```python
from build123d import *

# Parameters (mm, degrees)
F0_W     = 395
F0_H     = 121
F1_DEPTH = 35.5
F2_W     = 120
F2_H     = 120
F3_DEPTH = 33
F4_R     = 10.191795
F5_DEPTH = 10
F6_R     = 2.5
F7_DEPTH = 10


with BuildPart() as f1:
    # F0 (on Right) → F1 (new body)
    with BuildSketch(Plane.YZ):
        Rectangle(F0_W, F0_H)
    extrude(amount=F1_DEPTH)

    # F2 (on face) → F3 (join)
    with BuildSketch(Plane(origin=(0, 0, 0), x_dir=(0, -1, 0), z_dir=(-1, 0, 0))):
        with Locations((-134.5, 0)):
            Rectangle(F2_W, F2_H)
        with Locations((-11.5, 0)):
            Rectangle(F2_W, F2_H)
        with Locations((111.5, 0)):
            Rectangle(F2_W, F2_H)
    extrude(amount=F3_DEPTH)

    # F4 (on face) → F5 (join)
    with BuildSketch(Plane(origin=(0, 0, 0), x_dir=(0, -1, 0), z_dir=(-1, 0, 0))):
        with Locations((185, 45)):
            Circle(F4_R)
        with Locations((185, -45)):
            Circle(F4_R)
    extrude(amount=F5_DEPTH)

    # F6 (on face) → F7 (cut)
    with BuildSketch(Plane.YZ.offset(35.5)):
        with Locations((180.5, -52.5)):
            Circle(F6_R)
        with Locations((75.5, -52.5)):
            Circle(F6_R)
        with Locations((60.5, -52.5)):
            Circle(F6_R)
        with Locations((180.5, 52.5)):
            Circle(F6_R)
        with Locations((75.5, 52.5)):
            Circle(F6_R)
        with Locations((60.5, 52.5)):
            Circle(F6_R)
        with Locations((-44.5, 52.5)):
            Circle(F6_R)
        with Locations((-59.5, 52.5)):
            Circle(F6_R)
        with Locations((-164.5, 52.5)):
            Circle(F6_R)
        with Locations((-44.5, -52.5)):
            Circle(F6_R)
        with Locations((-164.5, -52.5)):
            Circle(F6_R)
        with Locations((-59.5, -52.5)):
            Circle(F6_R)
    extrude(amount=-F7_DEPTH, mode=Mode.SUBTRACT)


solid = f1.part
```
Geometry check sheet. Reference: the model listing, model coordinates, mm. A direction names the side the tool comes from. Round coordinates to 2 decimals unless told otherwise and drop trailing zeros. Loops run counter-clockwise (first coordinate to the right, second up) from the corner with the lowest first, then second, coordinate; pieces in that order, holes last. Notation, with made-up numbers: (0.5, -16) - (5.5, -16) arc R24 ccw to (5.5, 15) - close; hole circle Ø4 at (84, 57). An arc over 180 degrees is marked (long way). Write item = value, one per line. Start each with the question number.
1. Set-up check for faces 1 (the face through (-16, 71.5, -1)), 2 (the face through (-10, -185, -45)), 3 (the face through (-4.93, -174.82, -44.55)): record each of +Z, -Z, +X, -X, +Y, -Y from which the full face is reachable in a straight line by a thin tool's end or side.
2. Depth check by flat-ended pin: pin 1 (2.5 mm diameter, centred on y = -165, z = 51.5, fed in from +X); pin 2 (16.5 mm diameter, centred on x = -15.5, z = 1.5, fed in from +Y); pin 3 (5.5 mm diameter, centred on y = -58.5, z = 52, fed in from +X); pin 4 (16.5 mm diameter, centred on x = -20.5, y = -132, fed in from -Z). Enter the tip coordinate at first touch or a pass-through.
3. Thickness scan on line 1 (Y direction, x = -30, z = 7); line 2 (Z direction, x = 33, y = 75); line 3 (Z direction, x = 29.5, y = -164.5). Record the ranges inside material, lowest first.
4. Mould release check, pull along Y, two halves, no side actions. Record for faces 4 (the face through (0, -176, 0)), 5 (the face through (-16, 135, -60)): released by +Y, released by -Y, zero draft, split by the parting line, or undercut.
5. Section check B-B on z = -3. Enter the section's corners in (x, y).
6. Section check A-A on x = -6. Enter the section's corners in (y, z).
Working result:
q1.face_1 = +Z, -Z, -X
q1.face_2 = +Z, -Z, -X, -Y
q1.face_3 = -X
q2.pin_1 = 25.5
q2.pin_2 = 194.5
q2.pin_3 = 35.5
q2.pin_4 = -60
q3.line_1 = -171.5 to -51.5, -48.5 to 71.5, 74.5 to 194.5
q3.line_2 = -60.5 to -54.95, -50.05 to 50.05, 54.95 to 60.5
q3.line_3 = -60.5 to -55, -50 to 50, 55 to 60.5
q4.face_4 = undercut
q4.face_5 = zero draft
q5.outline = (-33, -171.5) - (0, -171.5) - (0, -197.5) - (35.5, -197.5) - (35.5, 197.5) - (0, 197.5) - (0, 194.5) - (-33, 194.5) - (-33, 74.5) - (0, 74.5) - (0, 71.5) - (-33, 71.5) - (-33, -48.5) - (0, -48.5) - (0, -51.5) - (-33, -51.5) - close
q6.outline = circle Ø20.38 at (-185, -45); circle Ø20.38 at (-185, 45); (-171.5, -60) - (-51.5, -60) - (-51.5, 60) - (-171.5, 60) - close; (-48.5, -60) - (71.5, -60) - (71.5, 60) - (-48.5, 60) - close; (74.5, -60) - (194.5, -60) - (194.5, 60) - (74.5, 60) - close
